```python
from build123d import *

# Parameters (mm, degrees)
SKETCH1_R           = 9
SKETCH1_R_2         = 10
BOSS_EXTRUDE1_DEPTH = 50


with BuildPart() as part:
    # Sketch1 → Boss-Extrude1 (new body)
    with BuildSketch(Plane.YZ):
        with BuildLine():
            Line((-25, -16.583123952), (-25, -75))
            Line((-25, -75), (-5, -75))
            Line((-5, -75), (-5, -30))
            Line((-5, -30), (5, -30))
            Line((5, -30), (5, -75))
            Line((5, -75), (25, -75))
            Line((25, -75), (25, -16.583123952))
            ThreePointArc((25, -16.583123952), (26.602160846, -13.868130311), (27.910571474, -11))
            Line((27.910571474, -11), (72.089428526, -11))
            ThreePointArc((72.089428526, -11), (130, 0), (72.089428526, 11))
            Line((72.089428526, 11), (27.910571474, 11))
            ThreePointArc((27.910571474, 11), (-13.868130311, 26.602160846), (-25, -16.583123952))
        make_face()
        with Locations(Location((0, 0, 0), (0, 0, 270))):
            Circle(SKETCH1_R, mode=Mode.SUBTRACT)
        with Locations(Location((100, 0, 0), (0, 0, 270))):
            Circle(SKETCH1_R_2, mode=Mode.SUBTRACT)
    extrude(amount=-BOSS_EXTRUDE1_DEPTH)


solid = part.part
```
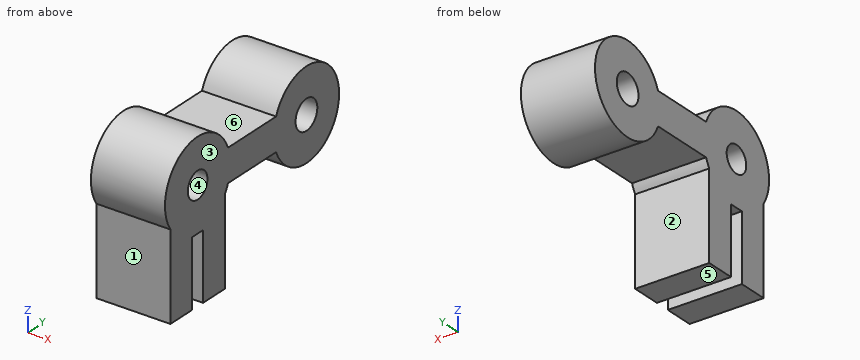
Here's how the part is built. I have some questions about the finished solid (model axes, mm). Face numbers are marked on the shaded views. A direction names the side the tool comes from. Coordinates: 2 decimals unless noted, no trailing zeros. Loops run counter-clockwise (first coordinate to the right, second up) from the corner with the lowest first, then second, coordinate; pieces in that order, holes last. Notation, with made-up numbers: (28, 59.25) -> (51, 59.25) arc R4 ccw to (51, 63.25) -> close; hole circle Ø5 at (79.5, -39.5). An arc over 180 degrees is marked (long way). Return JSON: item names as keys, results as strings.
1) I need wall thicknesses on line 1 (Y direction, x = -33, z = 0); line 2 (Y direction, x = -41, z = -1.5); line 3 (Z direction, x = -10, y = 57). Which ranges of each line are inside material? Lowest first, please. Write a range as from..to.
Results below:
{"line 1": "-30..-9, 9..90, 110..130", "line 2": "-29.96..-8.87, 8.87..90.11, 109.89..129.96", "line 3": "-11..11"}
2) Thinking about a two-plate mould opening in Z: for the marked faces 4, 5 and 6, which applies, +Z half, -Z half, draft (parallel to the pull), parting line (faces both ways), or undercut?
Results below:
{"face 4": "undercut", "face 5": "-Z half", "face 6": "+Z half"}
3) Will these pins go through, and if not, where does the flat tip stop? pin 1 (6 mm diameter, centred on x = -34.5, y = -9.5, fed in from +Z); pin 2 (13.5 mm diameter, centred on x = -34, z = -61.5, fed in from -Y); pin 3 (8 mm diameter, centred on x = -7, z = -11, fed in from -Y).
Results below:
{"pin 1": "z = 29.29", "pin 2": "y = -25", "pin 3": "y = -29.17"}
4) If we section it at C-C, the plane z = 0: Write out the boundary of the cut face in (x, y).
Results below:
{"outline": "(-50, -30) -> (0, -30) -> (0, -9) -> (-50, -9) -> close; (-50, 9) -> (0, 9) -> (0, 90) -> (-50, 90) -> close; (-50, 110) -> (0, 110) -> (0, 130) -> (-50, 130) -> close"}
5) If we section it at B-B, the plane y = 100: Write out the boundary of the cut face in (x, z), then the cut area to 3 significant figures.
Results below:
{"outline": "(-50, -30) -> (0, -30) -> (0, -10) -> (-50, -10) -> close; (-50, 10) -> (0, 10) -> (0, 30) -> (-50, 30) -> close", "area": "2,000 mm²"}
6) If we section it at A-A, the plane z = -39: Write out the boundary of the cut face in (x, y).
Results below:
{"outline": "(-50, -25) -> (0, -25) -> (0, -5) -> (-50, -5) -> close; (-50, 5) -> (0, 5) -> (0, 25) -> (-50, 25) -> close"}
7) For the marked faces 1, 2 and 3, which set-ups out of +Z, -Z, +X, -X, +Y, -Y let a thin tool reach every point of the face, with its end or its side?
Results below:
{"face 1": "-Z, +X, -X, -Y", "face 2": "-Z, +X, -X", "face 3": "+Z, -Z, +X, +Y, -Y"}
8) If we section it at D-D, the plane x = -19.5: Write out the boundary of the cut face in (y, z).
Results below:
{"outline": "(-25, -75) -> (-5, -75) -> (-5, -30) -> (5, -30) -> (5, -75) -> (25, -75) -> (25, -16.58) arc R30 ccw to (27.91, -11) -> (72.09, -11) arc R30 ccw (long way) to (72.09, 11) -> (27.91, 11) arc R30 ccw (long way) to (-25, -16.58) -> close; hole circle Ø18 at (0, 0); hole circle Ø20 at (100, 0)"}
